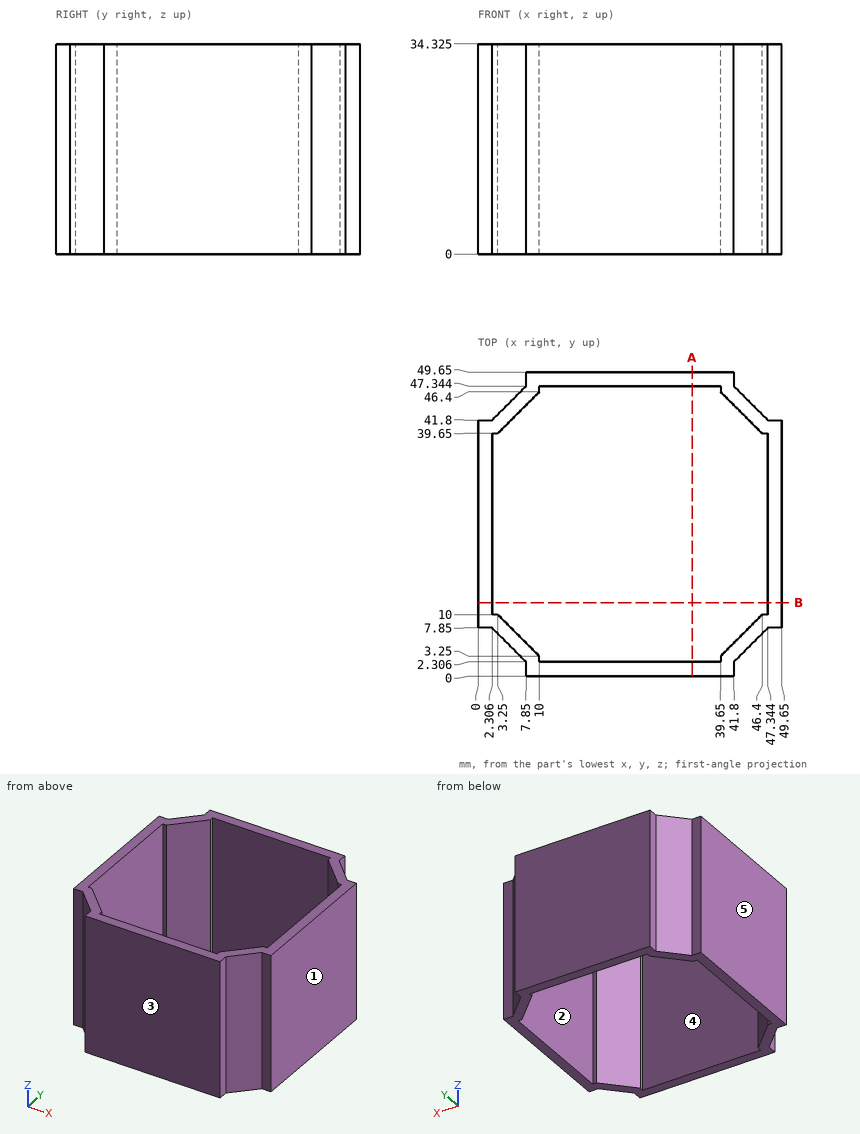
Input: dimensioned drawing with shaded views. Units: mm. Origin: part minimum x, y, z. A direction names the side the tool comes from. Round coordinates to 2 decimals unless told otherwise and drop trailing zeros. Loops run counter-clockwise (first coordinate to the right, second up) from the corner with the lowest first, then second, coordinate; pieces in that order, holes last. Notation, with made-up numbers: (23.25, 20.5) -> (57.25, 20.5) arc R28 cw to (57.25, 41.5) -> close; hole circle Ø2 at (80.5, -21.5). An arc over 180 degrees is marked (long way). Answer as a JSON object with one key per item and string values. Group by question number.
Q1. Mould query, pull axis Y, two halves, no side actions, for the marked faces 3, 4 and 5. Classes: pulls with the +Y half, pulls with the -Y half, needs draft (parallel to the pull), parting line crosses it, or undercut.
Q2. Contact query for flat-ended pins moving along their axis: P1, Ø3, axis at y = 11.5, z = 4, coming from the -X side; P2, Ø0.7, axis at y = 48.5, z = 14.5, coming from the -X side; P3, Ø0.8, axis at y = 47, z = 11, coming from the +X side; P4, Ø0.5, axis at y = 47, z = 17, coming from the -X side. Output: stop coordinate, or through.
Q3. Access query for the marked faces 1 and 2. Directions: +Z, -Z, +X, -X, +Y, -Y. A direction counts if a zero-diameter tool reaches every point of the face in a straight line with its end or side. Return the directions, or none.
Q4. Ray query, line 1 (Y direction, x = 36, z = 13); line 2 (Y direction, x = 5, z = 26). Return the intervals inside material, ascending. Write a range as from..to.
Q5. Section query A-A (x = 35). Output: boundary loops of the cut face in (y, z) (3 decimals).
Completed:
{
 "1": {"face 3": "pulls with the -Y half", "face 4": "undercut", "face 5": "needs draft"},
 "2": {"P1": "x = 0", "P2": "x = 7.85", "P3": "x = 42.54", "P4": "x = 7.26"},
 "3": {"face 1": "+Z, -Z, +X, +Y, -Y", "face 2": "+Z, -Z"},
 "4": {"line 1": "0..2.31, 47.34..49.65", "line 2": "5.16..8.25, 41.4..44.49"},
 "5": {"outline": "(0, 0) -> (2.306, 0) -> (2.306, 34.325) -> (0, 34.325) -> close; (47.344, 0) -> (49.65, 0) -> (49.65, 34.325) -> (47.344, 34.325) -> close"}
}
